```python
from build123d import *

# Parameters (mm, degrees)
F0_R     = 223.5
F1_DEPTH = 30
F2_SIZE  = 2
F3_R     = 40.75
F4_DEPTH = 30
F3_R_2   = 60
F3_R_3   = 3
F5_DEPTH = 8
F6_DEPTH = 30.001


with BuildPart() as f1:
    # F0 (on Top) → F1 (new body)
    with BuildSketch(Plane.XY):
        Circle(F0_R)
    extrude(amount=F1_DEPTH)

    # F2
    f2_edges = [f1.edges().sort_by_distance(p)[0] for p in [
        (-223.5, 0, 30),
        (-223.5, 0, 0),
    ]]
    chamfer(f2_edges, length=F2_SIZE)

    # F3 (on face) → F4 (cut)
    with BuildSketch(Plane.XY.offset(30)):
        Circle(F3_R)
    extrude(amount=-F4_DEPTH, mode=Mode.SUBTRACT)

    # F3 (on face) → F5 (cut)
    with BuildSketch(Plane.XY.offset(30)):
        Circle(F3_R_2)
        with Locations((-36.062446, -36.062446)):
            Circle(F3_R_3, mode=Mode.SUBTRACT)
        Circle(F3_R, mode=Mode.SUBTRACT)
        with Locations((36.062446, -36.062446)):
            Circle(F3_R_3, mode=Mode.SUBTRACT)
        with Locations((-36.062446, 36.062446)):
            Circle(F3_R_3, mode=Mode.SUBTRACT)
        with Locations((36.062446, 36.062446)):
            Circle(F3_R_3, mode=Mode.SUBTRACT)
        with Locations((-36.062446, 36.062446)):
            Circle(F3_R_3)
        with Locations((36.062446, 36.062446)):
            Circle(F3_R_3)
        with Locations((36.062446, -36.062446)):
            Circle(F3_R_3)
        with Locations((-36.062446, -36.062446)):
            Circle(F3_R_3)
    extrude(amount=-F5_DEPTH, mode=Mode.SUBTRACT)

    # F3 (on face) → F6 (cut, through all)
    with BuildSketch(Plane.XY.offset(30)):
        with Locations((-36.062446, 36.062446)):
            Circle(F3_R_3)
        with Locations((36.062446, 36.062446)):
            Circle(F3_R_3)
        with Locations((36.062446, -36.062446)):
            Circle(F3_R_3)
        with Locations((-36.062446, -36.062446)):
            Circle(F3_R_3)
    extrude(amount=-F6_DEPTH, mode=Mode.SUBTRACT)


solid = f1.part
```
Read the model definition and answer for the solid it produces. Units are mm, in the model's axes. A direction names the side the tool comes from. Round coordinates to 2 decimals unless told otherwise and drop trailing zeros. Write each loop counter-clockwise with the first axis right and the second up, starting at its lowest first coordinate (ties: lowest second). Pieces come first, ordered by that corner, then holes. Notation, with made-up numbers: (-38.5, 79) - (11.5, 79) arc R22 cw to (11.5, 113) - close; hole circle Ø1 at (10, 39). An arc over 180 degrees is marked (long way). One line per item, written item: value.
Q1. Find section A-A (y = 0). Determine the outline of the cut face in (x, z).
The answers:
outline: (-223.5, 2) - (-221.5, 0) - (-40.75, 0) - (-40.75, 22) - (-60, 22) - (-60, 30) - (-221.5, 30) - (-223.5, 28) - close; (40.75, 0) - (221.5, 0) - (223.5, 2) - (223.5, 28) - (221.5, 30) - (60, 30) - (60, 22) - (40.75, 22) - close
Q2. Which of the six approach directions +Z, -Z, +X, -X, +Y, -Y give full straight-line access (tool end or side, diameter ignored) to faces 1 (the flat face through (-3, -46, 0)), 2 (the cylindrical face through (-59.94, 2.64, 26.06))?
The answers:
face 1: -Z, +X, -X, +Y, -Y
face 2: +Z
Q3. For a pull along Y with two mould halves and no side action, classify faces 3 (the flat face through (12.5, -39.2, 22)), 4 (the flat face through (46, -46, 30)), 5 (the cylindrical face through (37.64, -15.61, 11.15)), 6 (the cylindrical face through (213.18, 67.13, 14.82)) as pulls with the +Y half, pulls with the -Y half, needs draft (parallel to the pull), parting line crosses it, or undercut.
The answers:
face 3: undercut
face 4: needs draft
face 5: undercut
face 6: parting line crosses it
Q4. Find section C-C (z = 14.5). Determine the outline of the cut face in (x, y), and give its area (3 significant figures).
The answers:
outline: circle Ø447 at (0, 0); hole circle Ø81.5 at (0, 0); hole circle Ø6 at (-36.06, -36.06); hole circle Ø6 at (-36.06, 36.06); hole circle Ø6 at (36.06, -36.06); hole circle Ø6 at (36.06, 36.06)
area: 152,000 mm2
Q5. Each of these flat-tipped pins is pushed along its axis until it touches: P1, Ø12, axis at y = 75, z = 26.5, coming from the -X side; P2, Ø10, axis at x = 155.5, z = 8, coming from the -Y side; P3, Ø3.5, axis at x = -36.06, y = 36.06, coming from the +Z side; P4, Ø6, axis at x = -14, z = 12, coming from the +Y side. Where does it stop, or does it pass through?
The answers:
P1: stops at x = -212.58
P2: stops at y = -165.23
P3: passes through
P4: stops at y = 223.23
Q6. Straight lines are drawn through the part: line 1 (Z direction, x = -25.5, y = -50.5); line 2 (Y direction, x = 0, z = 28); line 3 (Y direction, x = 7, z = 21.5). For each, find the intervals that lie inside material, in ascending order. Write a range as from..to.
The answers:
line 1: z = 0..22
line 2: y = -223.5..-60, 60..223.5
line 3: y = -223.39..-40.14, 40.14..223.39
